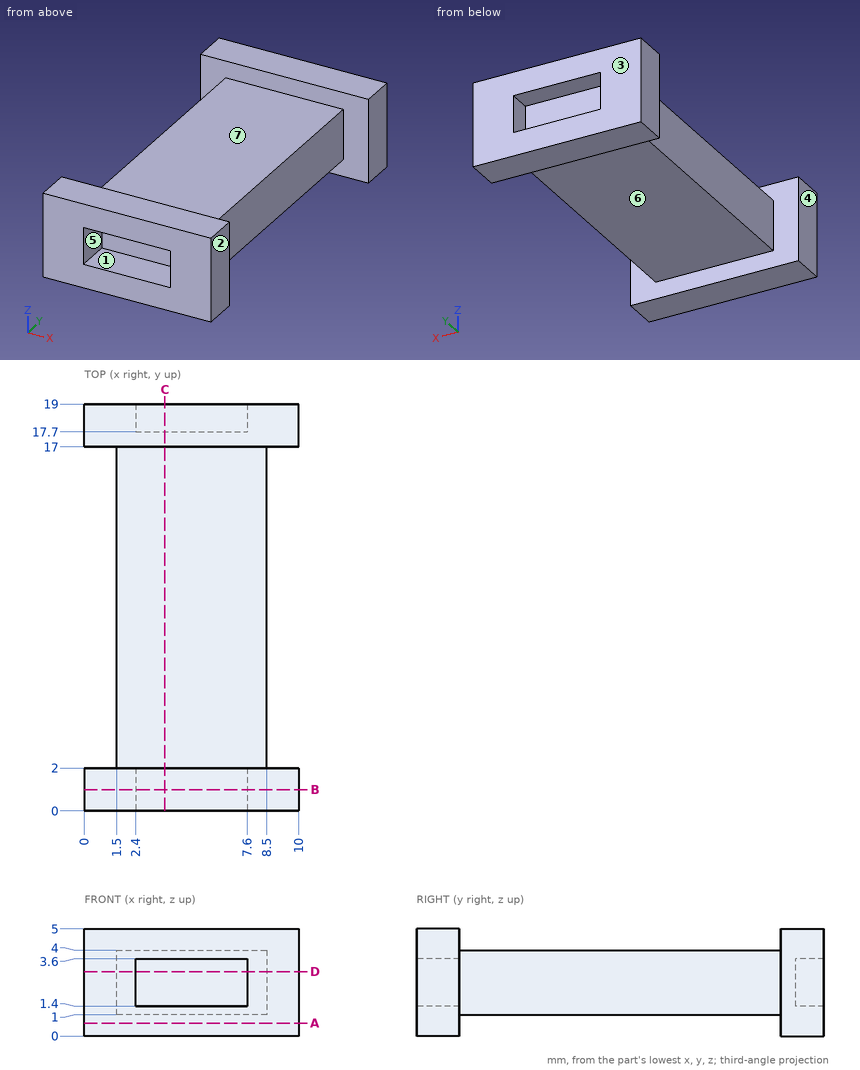
Drawing for the job (mm, zero at the part's lowest x, y, z). A direction names the side the tool comes from. Give positions to 0.01 mm unless a question says otherwise; leave off trailing zeros. Write each loop counter-clockwise with the first axis right and the second up, starting at its lowest first coordinate (ties: lowest second). Pieces come first, ordered by that corner, then holes. Notation, with made-up numbers: (-28, 48) -> (13, 48) arc R18 cw to (13, 59) -> close; hole circle Ø2 at (11, 83.25). An arc over 180 degrees is marked (long way). Put each result on its own line as item: value. Start each with the question number.
Item 1: Cut at C-C (x = 3.75). List the corners of the cut face in (y, z), then the cut area to 3 significant figures.
Item 2: Cut at D-D (z = 3). List the corners of the cut face in (x, y).
Item 3: Cut at B-B (y = 1). List the corners of the cut face in (x, z), then the cut area to 3 significant figures.
Item 4: Which spindle directions (+Z, -Z, +X, -X, +Y, -Y) get a long thin tool onto all of the face, cutting with end or side? Do the marked faces 5, 6 and 7. Say none if no direction does.
Item 5: Wall check: L1, parallel to Z at x = 4, y = 1; L2, parallel to Z at x = 7, y = 7.5; L3, parallel to Y at x = 6.75, z = 0.55. Give the ranges that are in metal, low to high. Write a range as [from, to].
Item 6: Cut at A-A (z = 0.6). List the corners of the cut face in (x, y).
Item 7: Pin check, flat tips, straight feed: pin 1 Ø2.5 at (x, z) = (4, 2.5) entering from -Y; pin 2 Ø2 at (y, z) = (14, 1) entering from +X; pin 3 Ø1 at (x, y) = (5.5, 13.5) entering from -Z; pin 4 Ø1.1 at (x, z) = (5.5, 2) entering from +Y. Stop position of each tip, or through.
Item 8: Pull direction X, two halves, no side cores. Call the marked faces 1, 2, 3 and 4: pulls with the +X half, pulls with the -X half, needs draft (parallel to the pull), parting line crosses it, or undercut.
Answer list:
1. outline: (0, 0) -> (2, 0) -> (2, 1) -> (17, 1) -> (17, 0) -> (19, 0) -> (19, 1.4) -> (17.7, 1.4) -> (17.7, 3.6) -> (19, 3.6) -> (19, 5) -> (17, 5) -> (17, 4) -> (2, 4) -> (2, 5) -> (0, 5) -> (0, 3.6) -> (2, 3.6) -> (2, 1.4) -> (0, 1.4) -> close
1. area: 57.7 mm2
2. outline: (0, 0) -> (2.4, 0) -> (2.4, 2) -> (7.6, 2) -> (7.6, 0) -> (10, 0) -> (10, 2) -> (8.5, 2) -> (8.5, 17) -> (10, 17) -> (10, 19) -> (7.6, 19) -> (7.6, 17.7) -> (2.4, 17.7) -> (2.4, 19) -> (0, 19) -> (0, 17) -> (1.5, 17) -> (1.5, 2) -> (0, 2) -> close
3. outline: (0, 0) -> (10, 0) -> (10, 5) -> (0, 5) -> close; hole (2.4, 1.4) -> (7.6, 1.4) -> (7.6, 3.6) -> (2.4, 3.6) -> close
3. area: 38.6 mm2
4. face 5: -Y
4. face 6: -Z, +X, -X
4. face 7: +Z, +X, -X
5. L1: z = [0, 1.4], [3.6, 5]
5. L2: z = [1, 4]
5. L3: y = [0, 2], [17, 19]
6. outline: (0, 0) -> (10, 0) -> (10, 2) -> (0, 2) -> close; (0, 17) -> (10, 17) -> (10, 19) -> (0, 19) -> close
7. pin 1: stops at y = 0
7. pin 2: stops at x = 8.5
7. pin 3: stops at z = 1
7. pin 4: stops at y = 17.7
8. face 1: undercut
8. face 2: pulls with the +X half
8. face 3: needs draft
8. face 4: pulls with the -X half
